from build123d import *

# Parameters (mm, degrees)
SKETCH1_W                                           = 70
SKETCH1_H                                           = 70
BOSS_EXTRUDE1_DEPTH                                 = 10
SKETCH1_3_R                                         = 15
BOSS_EXTRUDE2_DEPTH                                 = 22.5
CUT_EXTRUDE1_START                                  = -1
SKETCH2_R                                           = 25.85
SKETCH2_R_2                                         = 15
CUT_EXTRUDE1_DEPTH                                  = 1
CBORE_FOR_M3_HEX_SOCKET_HEAD_CAP_SCREW1_D           = 3.6
CBORE_FOR_M3_HEX_SOCKET_HEAD_CAP_SCREW1_CBORE_D     = 6.5
CBORE_FOR_M3_HEX_SOCKET_HEAD_CAP_SCREW1_CBORE_DEPTH = 4.4
F_2_5MM_CHAMFER1_SIZE                               = 2.5
F_0_5MM_CHAMFER2_SIZE                               = 0.5


with BuildPart() as part:
    # Sketch1 → Boss-Extrude1 (new body)
    with BuildSketch(Plane(origin=(0, 0, 0), x_dir=(1, 0, 0), z_dir=(0, 1, 0))):
        Rectangle(SKETCH1_W, SKETCH1_H)
    extrude(amount=BOSS_EXTRUDE1_DEPTH)

    # Sketch1<3> → Boss-Extrude2 (add)
    with BuildSketch(Plane(origin=(0, 0, 0), x_dir=(1, 0, 0), z_dir=(0, 1, 0))):
        with Locations(Location((0, 0, 0), (0, 0, 270))):
            Circle(SKETCH1_3_R)
        with BuildLine():
            Line((-1.5, 2), (1.5, 2))
            ThreePointArc((1.5, 2), (0, -2.5), (-1.5, 2))
        make_face(mode=Mode.SUBTRACT)
    extrude(amount=-BOSS_EXTRUDE2_DEPTH)

    # Sketch2 → Cut-Extrude1 (cut)
    with BuildSketch(Plane.XZ.offset(CUT_EXTRUDE1_START)):
        with Locations(Location((0, 0, 0), (0, 0, 270))):
            Circle(SKETCH2_R)
        with Locations(Location((0, 0, 0), (0, 0, 90))):
            Circle(SKETCH2_R_2, mode=Mode.SUBTRACT)
    extrude(amount=CUT_EXTRUDE1_DEPTH, mode=Mode.SUBTRACT)

    # CBORE for M3 Hex Socket Head Cap Screw1 (through all)
    with Locations(Plane(origin=(0, 0, 0), x_dir=(-1, 0, 0), z_dir=(0, -1, 0))):
        with Locations((-28.5, 30.5), (28.5, -30.5), (-28.5, -30.5), (28.5, 30.5), (0, -30.5), (0, 30.5)):
            CounterBoreHole(CBORE_FOR_M3_HEX_SOCKET_HEAD_CAP_SCREW1_D / 2, CBORE_FOR_M3_HEX_SOCKET_HEAD_CAP_SCREW1_CBORE_D / 2, CBORE_FOR_M3_HEX_SOCKET_HEAD_CAP_SCREW1_CBORE_DEPTH)

    # 2,5mm Chamfer1
    f_2_5mm_chamfer1_edges = [part.edges().sort_by_distance(p)[0] for p in [
        (-35, 5, -35),
        (-35, 5, 35),
        (35, 5, 35),
        (35, 5, -35),
    ]]
    chamfer(f_2_5mm_chamfer1_edges, length=F_2_5MM_CHAMFER1_SIZE)

    # 0,5mm Chamfer2
    f_0_5mm_chamfer2_edges = [part.edges().sort_by_distance(p)[0] for p in [
        (0, -22.5, -2),
        (0, -22.5, -15),
        (0, -22.5, 2.5),
        (0, 0, 25.85),
        (3.25, 0, -30.5),
        (3.25, 0, 30.5),
        (-25.25, 0, -30.5),
        (31.75, 0, 30.5),
        (-25.25, 0, 30.5),
        (31.75, 0, -30.5),
        (0, 0, 35),
        (0, 0, -35),
        (35, 0, 0),
        (-35, 0, 0),
        (33.75, 0, -33.75),
        (-33.75, 0, -33.75),
        (33.75, 0, 33.75),
        (-33.75, 0, 33.75),
    ]]
    chamfer(f_0_5mm_chamfer2_edges, length=F_0_5MM_CHAMFER2_SIZE)


solid = part.part
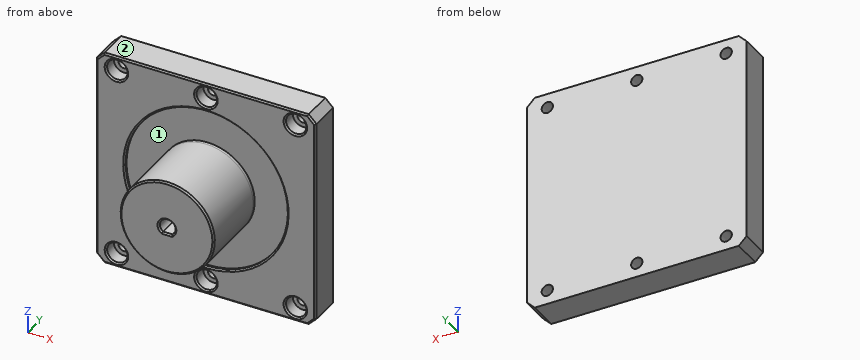
The listing builds one solid part. Answer for the finished solid, in the listing's coordinates (mm). Face numbers are marked on the shaded views. A direction names the side the tool comes from. Coordinates: 2 decimals unless noted, no trailing zeros. Write each loop counter-clockwise with the first axis right and the second up, starting at its lowest first coordinate (ties: lowest second). Pieces come first, ordered by that corner, then holes. Notation, with made-up numbers: (-25.5, -8) - (-11.5, -8) arc R23 ccw to (-11.5, 2) - close; hole circle Ø1 at (52, 8). An arc over 180 degrees is marked (long way). Return JSON: item names as keys, results as strings.
1. The part is cut by section C-C on z = 30.5. Count the separate pieces of the cut face and the enclosed holes in it, then the cut area to 3 significant figures.
Final values:
{"separate pieces": "4", "enclosed holes": "0", "area": "553 mm^2"}
2. The part is cut by section D-D on y = -5. Determine the outline of the cut face in (x, z), then the cut area to 3 significant figures.
Final values:
{"outline": "circle Ø30 at (0, 0); hole (-1.5, -2) - (1.5, -2) arc R2.5 ccw (long way) to start", "area": "688 mm^2"}
3. Each of these flat-tipped pins is pushed along its axis until it touches: pin 1 Ø1.5 at (x, y) = (0, -13) entering from +Z; pin 2 Ø7 at (x, z) = (27.5, -31) entering from -Y; pin 3 Ø1.5 at (x, z) = (11.5, -10.5) entering from -Y. Where does it stop, or does it pass through?
Final values:
{"pin 1": "z = 15", "pin 2": "y = 0", "pin 3": "y = -22.18"}
4. Consider line 1 along Z through (x, y) = (28.5, 8.65); line 2 along X through (y, z) = (2.05, 30.5); line 3 along X through (y, z) = (7.9, -30.5). Determine where each line is inside the solid, lowest interval first.
Final values:
{"line 1": "-35 to -32.3, -28.7 to 28.7, 32.3 to 35", "line 2": "-35 to -31.75, -25.25 to -3.25, 3.25 to 25.25, 31.75 to 35", "line 3": "-35 to -30.3, -26.7 to -1.8, 1.8 to 26.7, 30.3 to 35"}
5. The part is cut by section B-B on x = 28.5. Determine the outline of the cut face in (y, z).
Final values:
{"outline": "(0, -34.5) - (0.5, -35) - (10, -35) - (10, -32.3) - (4.4, -32.3) - (4.4, -33.75) - (0.5, -33.75) - (0, -34.25) - close; (0, -26.75) - (0.5, -27.25) - (4.4, -27.25) - (4.4, -28.7) - (10, -28.7) - (10, 28.7) - (4.4, 28.7) - (4.4, 27.25) - (0.5, 27.25) - (0, 26.75) - close; (0, 34.25) - (0.5, 33.75) - (4.4, 33.75) - (4.4, 32.3) - (10, 32.3) - (10, 35) - (0.5, 35) - (0, 34.5) - close"}
6. Which of the six approach directions +Z, -Z, +X, -X, +Y, -Y give full straight-line access (tool end or side, diameter ignored) to the marked faces 1 and 2?
Final values:
{"face 1": "-Y", "face 2": "+Z, +X, -X, +Y, -Y"}
7. The part is cut by section A-A on z = 0. Determine the outline of the cut face in (x, y).
Final values:
{"outline": "(-35, 0.5) - (-34.5, 0) - (-26.35, 0) - (-25.85, 0.5) - (-25.85, 1) - (-15, 1) - (-15, -22) - (-14.5, -22.5) - (-3, -22.5) - (-2.5, -22) - (-2.5, 0) - (2.5, 0) - (2.5, -22) - (3, -22.5) - (14.5, -22.5) - (15, -22) - (15, 1) - (25.85, 1) - (25.85, 0.5) - (26.35, 0) - (34.5, 0) - (35, 0.5) - (35, 10) - (-35, 10) - close"}
